```python
from build123d import *

# Parameters (mm, degrees)
SKETCH_1_W                   = 26
SKETCH_1_H                   = 7
EXTRUDE_1_DEPTH              = 36
CUT_EXTRUDE_1_DEPTH          = 45.544921147
HOLE_WIZARD_M32_D            = 2.5
HOLE_WIZARD_M32_DEPTH        = 5
HOLE_WIZARD_M32_CSINK_D      = 3.55
HOLE_WIZARD_M32_CSINK_ANGLE  = 90
HOLE_WIZARD_M33_D            = 2.5
HOLE_WIZARD_M33_DEPTH        = 5
HOLE_WIZARD_M33_CSINK_D      = 3.55
HOLE_WIZARD_M33_CSINK_ANGLE  = 90
CUT_EXTRUDE_4_DEPTH          = 39.910152917
HOLE_WIZARD_M31_9_AT_2_COUNT = 2
HOLE_WIZARD_M31_9_AT_2_PITCH = 8


# Read off the part's stored shape, not the designer's step: Отверстие обработанное метчиком M31
with BuildPart() as part:
    # Эскиз1 → Бобышка-Вытянуть1 (new body)
    with BuildSketch(Plane(origin=(0, 0, 0), x_dir=(1, 0, 0), z_dir=(0, 1, 0))):
        Rectangle(SKETCH_1_W, SKETCH_1_H)
    extrude(amount=EXTRUDE_1_DEPTH)

    # Эскиз2 → Вырез-Вытянуть1 (cut, through all)
    with BuildSketch(Plane.ZY.offset(13)):
        Polygon((-77.060994328, 31), (-3.5, 31), (1, 31), (1, 28.5), (-0.5, 28.5), (-0.5, 7.5), (1, 7.5), (1, 5), (-3.5, 5), (-77.060994328, 5), (-224.182982985, 5), (-224.182982985, 31), align=None)
    extrude(amount=-CUT_EXTRUDE_1_DEPTH, mode=Mode.SUBTRACT)

    # Hole Wizard M31 outline → Hole Wizard M31 (revolve, cut)
    with BuildSketch(Plane(origin=(10.5, 26, 0), x_dir=(1, 0, 0), z_dir=(0, -1, 0))):
        Polygon((0, -0.5), (1.775, -0.5), (1.25, 0.025), (1.25, 2.975), (1.775, 3.5), (0, 3.5), align=None)
    revolve(axis=Axis((10.5, 26, 0), (0, 0, 1)), mode=Mode.SUBTRACT)

    # Hole Wizard M31 2 outline → Hole Wizard M31 2 (revolve, cut)
    with BuildSketch(Plane(origin=(-10.5, 10, 0), x_dir=(1, 0, 0), z_dir=(0, -1, 0))):
        Polygon((0, -0.5), (1.775, -0.5), (1.25, 0.025), (1.25, 2.975), (1.775, 3.5), (0, 3.5), align=None)
    revolve(axis=Axis((-10.5, 10, 0), (0, 0, 1)), mode=Mode.SUBTRACT)

    # Hole Wizard M31 3 outline → Hole Wizard M31 3 (revolve, cut)
    with BuildSketch(Plane(origin=(-10.5, 26, 0), x_dir=(1, 0, 0), z_dir=(0, -1, 0))):
        Polygon((0, -0.5), (1.775, -0.5), (1.25, 0.025), (1.25, 2.975), (1.775, 3.5), (0, 3.5), align=None)
    revolve(axis=Axis((-10.5, 26, 0), (0, 0, 1)), mode=Mode.SUBTRACT)

    # Hole Wizard M31 4 outline → Hole Wizard M31 4 (revolve, cut)
    with BuildSketch(Plane(origin=(10.5, 10, 0), x_dir=(1, 0, 0), z_dir=(0, -1, 0))):
        Polygon((0, -0.5), (1.775, -0.5), (1.25, 0.025), (1.25, 2.975), (1.775, 3.5), (0, 3.5), align=None)
    revolve(axis=Axis((10.5, 10, 0), (0, 0, 1)), mode=Mode.SUBTRACT)

    # Hole Wizard M31 5 outline → Hole Wizard M31 5 (revolve, cut)
    with BuildSketch(Plane(origin=(-3, 33, 0), x_dir=(1, 0, 0), z_dir=(0, -1, 0))):
        Polygon((0, -3.5), (1.775, -3.5), (1.25, -2.975), (1.25, 2.975), (1.775, 3.5), (0, 3.5), align=None)
    revolve(axis=Axis((-3, 33, 0), (0, 0, 1)), mode=Mode.SUBTRACT)

    # Hole Wizard M31 6 outline → Hole Wizard M31 6 (revolve, cut)
    with BuildSketch(Plane(origin=(3, 3, 0), x_dir=(1, 0, 0), z_dir=(0, -1, 0))):
        Polygon((0, -3.5), (1.775, -3.5), (1.25, -2.975), (1.25, 2.975), (1.775, 3.5), (0, 3.5), align=None)
    revolve(axis=Axis((3, 3, 0), (0, 0, 1)), mode=Mode.SUBTRACT)

    # Hole Wizard M31 7 outline → Hole Wizard M31 7 (revolve, cut)
    with BuildSketch(Plane(origin=(-3, 3, 0), x_dir=(1, 0, 0), z_dir=(0, -1, 0))):
        Polygon((0, -3.5), (1.775, -3.5), (1.25, -2.975), (1.25, 2.975), (1.775, 3.5), (0, 3.5), align=None)
    revolve(axis=Axis((-3, 3, 0), (0, 0, 1)), mode=Mode.SUBTRACT)

    # Hole Wizard M31 8 outline → Hole Wizard M31 8 (revolve, cut)
    with BuildSketch(Plane(origin=(3, 33, 0), x_dir=(1, 0, 0), z_dir=(0, -1, 0))):
        Polygon((0, -3.5), (1.775, -3.5), (1.25, -2.975), (1.25, 2.975), (1.775, 3.5), (0, 3.5), align=None)
    revolve(axis=Axis((3, 33, 0), (0, 0, 1)), mode=Mode.SUBTRACT)

    # Отверстие обработанное метчиком M32
    with Locations(Plane.XZ):
        with Locations((8, -0.5), (-8, -0.5)):
            CounterSinkHole(HOLE_WIZARD_M32_D / 2, HOLE_WIZARD_M32_CSINK_D / 2, depth=HOLE_WIZARD_M32_DEPTH, counter_sink_angle=HOLE_WIZARD_M32_CSINK_ANGLE)

    # Отверстие обработанное метчиком M33
    with Locations(Plane(origin=(0, 36, 0), x_dir=(-1, 0, 0), z_dir=(0, 1, 0))):
        with Locations((8, -0.5), (-8, -0.5)):
            CounterSinkHole(HOLE_WIZARD_M33_D / 2, HOLE_WIZARD_M33_CSINK_D / 2, depth=HOLE_WIZARD_M33_DEPTH, counter_sink_angle=HOLE_WIZARD_M33_CSINK_ANGLE)

    # Эскиз10 → Вырез-Вытянуть4 (cut, through all)
    with BuildSketch(Plane.XY.offset(3.5)):
        with BuildLine():
            ThreePointArc((-13, 14.127016654), (-10, 18), (-13, 21.872983346))
            Line((-13, 21.872983346), (-13, 14.127016654))
        make_face()
        with BuildLine():
            Line((13, 14.127016654), (13, 21.872983346))
            ThreePointArc((13, 21.872983346), (10, 18), (13, 14.127016654))
        make_face()
    extrude(amount=-CUT_EXTRUDE_4_DEPTH, mode=Mode.SUBTRACT)

    # Эскиз11 → Hole Wizard M31 9 (revolve, cut)
    with BuildSketch(Plane(origin=(-4, 18, 3.5), x_dir=(0, -1, 0), z_dir=(1, 0, 0))):
        Polygon((0, 0), (0, 4), (2.5, 4), (2.4, 3.9), (2.4, 3.1), (2.5, 3), (3.25, 3), (3.25, 0.1), (3.35, 0), align=None)
    hole_wizard_m31_9 = revolve(axis=Axis((-4, 18, 9.85), (0, 0, -1)), mode=Mode.SUBTRACT)

    # Hole Wizard M31 9 at 2: Hole Wizard M31 9 ×2
    with Locations(*[(i * HOLE_WIZARD_M31_9_AT_2_PITCH, 0, 0) for i in range(1, HOLE_WIZARD_M31_9_AT_2_COUNT)]):
        add(hole_wizard_m31_9, mode=Mode.SUBTRACT)


solid = part.part
```
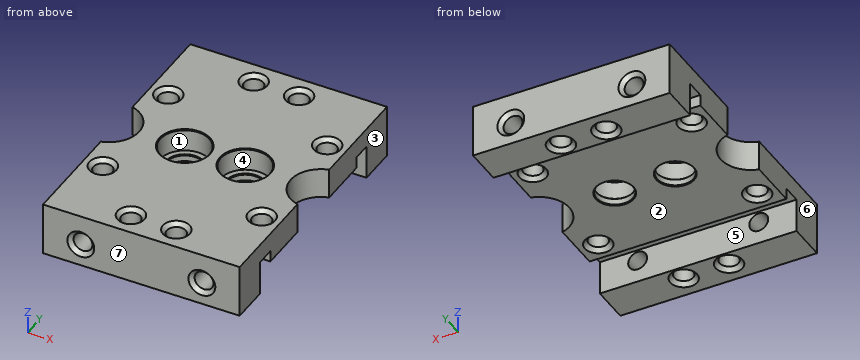
Read the model definition and answer for the solid it produces. Units are mm, in the model's axes. Face numbers are marked on the shaded views. A direction names the side the tool comes from. Give positions to 0.01 mm unless a question says otherwise; leave off trailing zeros. Order: outer loops, then holes, each group sorted by start corner. A loop starts at its lowest first (then second) coordinate and runs counter-clockwise, first axis right, second up. Notation, with made-up numbers: (50.25, -5.75) -> (94.25, -5.75) arc R23 cw to (94.25, 12.25) -> close; hole circle Ø10 at (-4, 72). An arc over 180 degrees is marked (long way). Write item = value, one per line.
1. Given pin 1 (2 mm diameter, centred on x = -8, z = -0.5, fed in from -Y); pin 2 (7.5 mm diameter, centred on x = -4, y = 18, fed in from -Z); pin 3 (3 mm diameter, centred on x = 3, y = 33, fed in from +Z) (3 decimals), each flat-ended and moving along its own axis, determine where each tip first touches the part or whether it passes through.
Numbers:
pin_1 = 7.5
pin_2 = -0.5
pin_3 = 3.225
2. A cutting plane is placed at C-C, the plane z = 2.5. Count the separate pieces of the cut face and the enclosed holes in it, and give its area (3 significant figures).
Numbers:
separate_pieces = 1
enclosed_holes = 10
area = 796 mm²
3. Straight lines are drawn through the part: line 1 along Y through (x, z) = (3, -0.55); line 2 along Y through (x, z) = (-0.25, 0); line 3 along X through (y, z) = (18, 2.85). For each, find the intervals that lie inside material, in ascending order.
Numbers:
line_1 = 0 to 1.75, 4.25 to 5, 31 to 31.75, 34.25 to 36
line_2 = 0 to 5, 7.5 to 28.5, 31 to 36
line_3 = -10 to -7.25, -0.75 to 0.75, 7.25 to 10
4. The mould has two halves that part along Y. Classify the marked faces 4, 5, 6 and 7: +Y half, -Y half, draft (parallel to the pull), parting line (faces both ways), or undercut.
Numbers:
face_4 = undercut
face_5 = undercut
face_6 = draft
face_7 = -Y half
5. A cutting plane is placed at A-A, the plane y = 3. Write down the section's boundary in (x, z) (3 decimals), and give its area (3 significant figures).
Numbers:
outline = (-13, -3.5) -> (-4.775, -3.5) -> (-4.25, -2.975) -> (-4.25, 2.975) -> (-4.775, 3.5) -> (-13, 3.5) -> close; (-1.75, -2.975) -> (-1.225, -3.5) -> (1.225, -3.5) -> (1.75, -2.975) -> (1.75, 2.975) -> (1.225, 3.5) -> (-1.225, 3.5) -> (-1.75, 2.975) -> close; (4.25, -2.975) -> (4.775, -3.5) -> (13, -3.5) -> (13, 3.5) -> (4.775, 3.5) -> (4.25, 2.975) -> close; hole circle Ø2.5 at (-8, -0.5); hole circle Ø2.5 at (8, -0.5)
area = 136 mm²
6. A cutting plane is placed at B-B, the plane x = -8. Write down the section's boundary in (y, z) (3 decimals).
Numbers:
outline = (0, -3.5) -> (5, -3.5) -> (5, -1.75) -> (0.525, -1.75) -> (0, -2.275) -> close; (0, 1.275) -> (0.525, 0.75) -> (5, 0.75) -> (5, 1) -> (7.5, 1) -> (7.5, -0.5) -> (28.5, -0.5) -> (28.5, 1) -> (31, 1) -> (31, 0.75) -> (35.475, 0.75) -> (36, 1.275) -> (36, 3.5) -> (0, 3.5) -> close; (31, -3.5) -> (36, -3.5) -> (36, -2.275) -> (35.475, -1.75) -> (31, -1.75) -> close
7. For the marked faces 1, 2 and 3, determine the directions among +Z, -Z, +X, -X, +Y, -Y from which every point of the face is accessible in a straight line to the end or side of a thin tool.
Numbers:
face_1 = +Z
face_2 = -Z, +X, -X
face_3 = +Z, -Z, +X, +Y, -Y
